Work out the finished part from the listing and answer in its coordinate system (mm). Round coordinates to 2 decimals unless told otherwise and drop trailing zeros. Loops run counter-clockwise (first coordinate to the right, second up) from the corner with the lowest first, then second, coordinate; pieces in that order, holes last. Notation, with made-up numbers: (25.25, 42) -> (83.25, 42) arc R19 cw to (83.25, 66) -> close; hole circle Ø1 at (-9, 71). An arc over 180 degrees is marked (long way). Use one line per item in the form item = value.
```python
from build123d import *

# Parameters (mm, degrees)
F0_W     = 6.096
F0_H     = 5.08
F1_DEPTH = 3.06


with BuildPart() as f1:
    # F0 (on Front) → F1 (new body)
    with BuildSketch(Plane.XZ):
        Polygon((-64.67925, -18.20163), (-60.735819, -18.20163), (-58.351868, -28.077984), (-54.011868, -28.077984), (-56.395819, -18.20163), (-76.14853, 40.42821), (-78.907189, 40.42821), (-85.003189, 40.42821), (-87.727705, 40.42821), align=None)
        with Locations((-81.955189, 42.96821)):
            Rectangle(F0_W, F0_H)
    extrude(amount=F1_DEPTH)


solid = f1.part
```
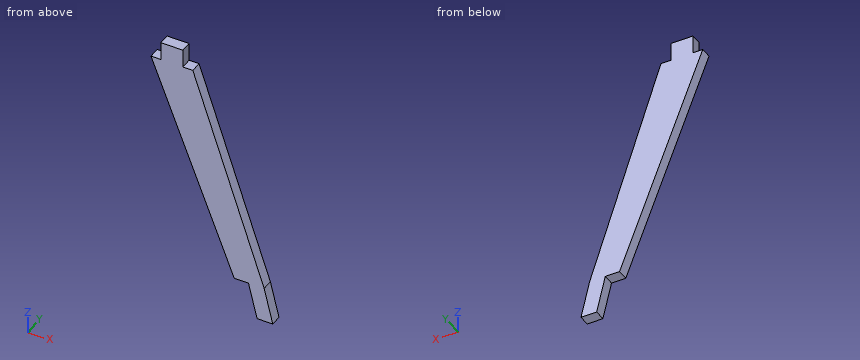
(1) Find section A-A, the plane y = -2.35. Write down the section's boundary in (x, z), then the cut area to 3 significant figures.
Completed:
outline = (-87.73, 40.43) -> (-64.68, -18.2) -> (-60.74, -18.2) -> (-58.35, -28.08) -> (-54.01, -28.08) -> (-56.4, -18.2) -> (-76.15, 40.43) -> (-78.91, 40.43) -> (-78.91, 45.51) -> (-85, 45.51) -> (-85, 40.43) -> close
area = 656 mm2
(2) Consider L1, parallel to X at y = -2.9, z = 38.5; L2, parallel to X at y = -2.5, z = -4.5. Determine where each line is inside the solid, lowest interval first.
Completed:
L1 = -86.97 to -75.5
L2 = -70.07 to -61.01
(3) Given P1, Ø0.8, axis at x = -86.5, y = -1.5, coming from the +Z side; P2, Ø0.9, axis at y = -1, z = 43.5, coming from the -X side; P3, Ø1.5, axis at y = -1.5, z = 19, coming from the -X side, each flat-ended and moving along its own axis, determine where each tip first touches the part or whether it passes through.
Completed:
P1 = 40.43
P2 = -85
P3 = -79.6
(4) Find section B-B, the plane z = 35. Write down the section's boundary in (x, y).
Completed:
outline = (-85.59, -3.06) -> (-74.32, -3.06) -> (-74.32, 0) -> (-85.59, 0) -> close
(5) Find section C-C, the plane x = -66. Write down the section's boundary in (y, z), then the cut area to 3 significant figures.
Completed:
outline = (-3.06, -14.84) -> (0, -14.84) -> (0, 10.31) -> (-3.06, 10.31) -> close
area = 77.0 mm2
